Design review of the part shown in the three views and the two pictorial views. Dimensions are in mm from the part's minimum x, y and z. A direction names the side the tool comes from. Coordinates: 2 decimals unless noted, no trailing zeros. Loops run counter-clockwise (first coordinate to the right, second up) from the corner with the lowest first, then second, coordinate; pieces in that order, holes last.
Q1. Add section B-B on x = 10. Give the boundary of the cut face in (y, z).
Q2. Draft analysis for pull direction X (two halves, no side actions). For the marked faces 1, 2 and 3, state which applies: released by +X, released by -X, zero draft, split by the parting line, or undercut.
Q3. Add section A-A on z = 16.5. Give the boundary of the cut face in (x, y).
Q4. Add section D-D on z = 10. Give the boundary of the cut face in (x, y).
Q5. Wall thickness on probe 1 along Y at (x, z) = (100, 1.7); probe 2 along Y at (x, z) = (24.35, 10); probe 3 along X at (y, z) = (46, 5.5): over which ranges is each line inside the solid? List them lowest first.
Q6. Machinability: for the marked faces 4, 5, 6, 7 and 8, which of the approach directions +Z, -Z, +X, -X, +Y, -Y give a long, thin tool a straight path to every point of the face, cutting with its end or side? Answer none if there is none.
Q7. For P1, Ø5, axis at x = 10, y = 25, coming from the -Z side; P2, Ø25, axis at x = 54.5, y = 27.5, coming from the -Z side; P3, Ø4.5, axis at x = 98, y = 34.5, coming from the +Z side; P4, Ø1.5, axis at y = 9.5, z = 13.5, coming from the +X side, all flat-tipped, find the tip position at first contact; note any pin that passes through.
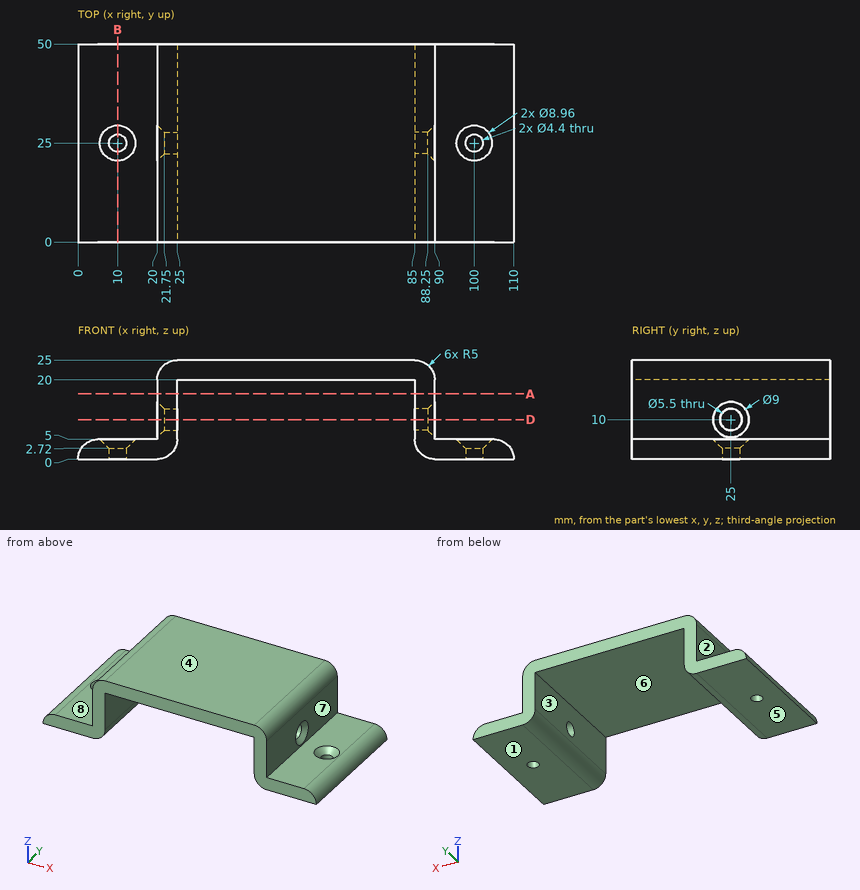
Entries:
1. outline: (0, 0) - (22.8, 0) - (22.8, 2.72) - (20.52, 5) - (0, 5) - close; (27.2, 0) - (50, 0) - (50, 5) - (29.48, 5) - (27.2, 2.72) - close
2. face 1: zero draft
2. face 2: released by -X
2. face 3: undercut
3. outline: (20, 0) - (25, 0) - (25, 50) - (20, 50) - close; (85, 0) - (90, 0) - (90, 50) - (85, 50) - close
4. outline: (20, 0) - (25, 0) - (25, 22.25) - (21.75, 22.25) - (20, 20.5) - close; (20, 29.5) - (21.75, 27.75) - (25, 27.75) - (25, 50) - (20, 50) - close; (85, 0) - (90, 0) - (90, 20.5) - (88.25, 22.25) - (85, 22.25) - close; (85, 27.75) - (88.25, 27.75) - (90, 29.5) - (90, 50) - (85, 50) - close
5. probe 1: y = 0 to 22.8, 27.2 to 50
5. probe 2: y = 0 to 22.25, 27.75 to 50
5. probe 3: x = 20 to 25, 85 to 90
6. face 4: +Z, +X, -X, +Y, -Y
6. face 5: -Z, +X, -X, +Y, -Y
6. face 6: -Z, +Y, -Y
6. face 7: +Z, +X, +Y, -Y
6. face 8: +Z, -X, +Y, -Y
7. P1: stops at z = 0
7. P2: stops at z = 20
7. P3: stops at z = 5
7. P4: stops at x = 90
